Build history of the part. All positions in model axes, mm. A direction names the side the tool comes from. Round coordinates to 2 decimals unless told otherwise and drop trailing zeros. Loops run counter-clockwise (first coordinate to the right, second up) from the corner with the lowest first, then second, coordinate; pieces in that order, holes last. Notation, with made-up numbers: (31, 19.5) -> (40, 19.5) arc R14 ccw to (40, 41.5) -> close; hole circle Ø11 at (54.5, 49.25). An arc over 180 degrees is marked (long way). Put each result on its own line as item: value. Start each with the question number.
Item 1: Tool access for faces 1 (the flat face through (6, 197, 0)), 2 (the cylindrical face through (2.71, 394.26, -6.74)): list every direction of +Z, -Z, +X, -X, +Y, -Y with a clear straight run to the whole face (end or side of a thin tool).
Item 2: Pull direction Y, two halves, no side cores. Call faces 3 (the flat face through (-7, 0, 0)), 4 (the cylindrical face through (2.71, 394.26, 6.76)), 5 (the flat face through (7.5, 197, 0)), 6 (the flat face through (-7, 400, 0)): +Y half, -Y half, draft (parallel to the pull), parting line (faces both ways), or undercut.
Item 3: Drill centre lines: probe 1 along Y at (x, z) = (0, 6.65); probe 2 along X at (y, z) = (50, -1.75); probe 3 along X at (y, z) = (370, 6.4). Where is each one in solid material? Low to high. Write a range as [from, to].
Item 4: Flat gauge pin, fed straight in: pin 1 Ø2.5 at (x, y) = (0, 370) entering from -Z. Where does the tip first touch, or does it go through?
Item 5: Cut at A-A, the plane y = 278. List the corners of the cut face in (x, z), plus the area to 3 significant figures.
```python
from build123d import *

# Parameters (mm, degrees)
SKETCH_1_W          = 15
SKETCH_1_H          = 15
SKETCH_1_W_2        = 12
SKETCH_1_H_2        = 12
EXTRUDE_1_DEPTH     = 400
SKETCH_2_R          = 5.05
SKETCH_2_R_2        = 1.6
CUT_EXTRUDE_1_DEPTH = 401.35140814
SKETCH_3_R          = 2.1
CUT_EXTRUDE_2_DEPTH = 401.35140814
SKETCH_4_R          = 3.1
CUT_EXTRUDE_3_DEPTH = 401.35140814
SKETCH_5_R          = 3.1
SKETCH_5_R_2        = 1.6
CUT_EXTRUDE_4_DEPTH = 401.35140814


with BuildPart() as part:
    # ｽｹｯﾁ1 → 押し出し-薄板1 (new body)
    with BuildSketch(Plane(origin=(0, 0, 0), x_dir=(1, 0, 0), z_dir=(0, 1, 0))):
        Rectangle(SKETCH_1_W, SKETCH_1_H)
        Rectangle(SKETCH_1_W_2, SKETCH_1_H_2, mode=Mode.SUBTRACT)
    extrude(amount=EXTRUDE_1_DEPTH)

    # ｽｹｯﾁ2 → ｶｯﾄ - 押し出し1 (cut, through all)
    with BuildSketch(Plane.XY.offset(7.5)):
        with Locations((0, 390)):
            Circle(SKETCH_2_R)
        with Locations((0, 370)):
            Circle(SKETCH_2_R_2)
    extrude(amount=-CUT_EXTRUDE_1_DEPTH, mode=Mode.SUBTRACT)

    # ｽｹｯﾁ3 → ｶｯﾄ - 押し出し2 (cut, through all)
    with BuildSketch(Plane(origin=(7.5, 0, 0), x_dir=(0, 0, -1), z_dir=(1, 0, 0))):
        with Locations((0, 390)):
            Circle(SKETCH_3_R)
    extrude(amount=-CUT_EXTRUDE_2_DEPTH, mode=Mode.SUBTRACT)

    # ｽｹｯﾁ4 → ｶｯﾄ - 押し出し3 (cut, through all)
    with BuildSketch(Plane(origin=(7.5, 0, 0), x_dir=(0, 0, -1), z_dir=(1, 0, 0))):
        with Locations((0, 5)):
            Circle(SKETCH_4_R)
    extrude(amount=-CUT_EXTRUDE_3_DEPTH, mode=Mode.SUBTRACT)

    # ｽｹｯﾁ5 → ｶｯﾄ - 押し出し4 (cut, through all)
    with BuildSketch(Plane(origin=(7.5, 0, 0), x_dir=(0, 0, -1), z_dir=(1, 0, 0))):
        with Locations((0, 5)):
            Circle(SKETCH_5_R)
        with Locations((0, 20)):
            Circle(SKETCH_5_R_2)
    extrude(amount=-CUT_EXTRUDE_4_DEPTH, mode=Mode.SUBTRACT)


solid = part.part
```
Reply:
1. face 1: +Y, -Y
1. face 2: +Z, -Z
2. face 3: -Y half
2. face 4: undercut
2. face 5: draft
2. face 6: +Y half
3. probe 1: y = [0, 368.4], [371.6, 384.95], [395.05, 400]
3. probe 2: x = [-7.5, -6], [6, 7.5]
3. probe 3: x = [-7.5, -1.6], [1.6, 7.5]
4. pin 1: passes through
5. outline: (-7.5, -7.5) -> (7.5, -7.5) -> (7.5, 7.5) -> (-7.5, 7.5) -> close; hole (-6, -6) -> (6, -6) -> (6, 6) -> (-6, 6) -> close
5. area: 81.0 mm^2
